Check sheet for the modelled part. Datum: model origin and axes. Units: mm. Face numbers are marked on the shaded views. A direction names the side the tool comes from. Give positions to 0.01 mm unless a question says otherwise; leave off trailing zeros. Order: outer loops, then holes, each group sorted by start corner. A loop starts at its lowest first (then second) coordinate and runs counter-clockwise, first axis right, second up.
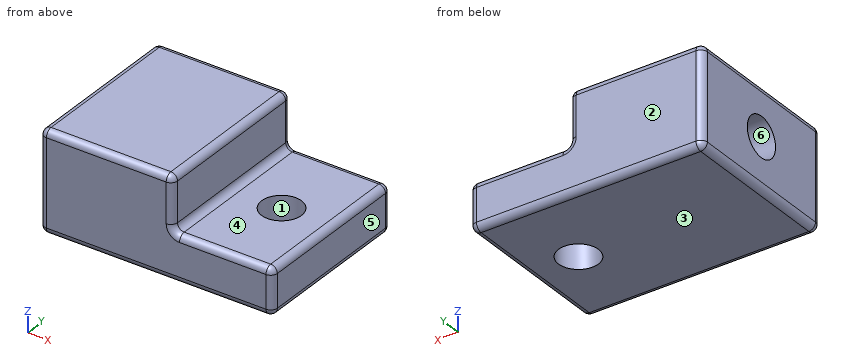
Autodesk Inventor part; units mm, degrees
ref_plane "YZ Plane" through (0, 0, 0) normal (1, 0, 0) x (0, 1, 0)
ref_plane "XZ Plane" through (0, 0, 0) normal (0, 1, 0) x (-1, 0, 0)
ref_plane "XY Plane" through (0, 0, 0) normal (0, 0, 1) x (1, 0, 0)
sketch "Boceto1" plane through (0, 0, 0) normal (0, 0, 1) x (1, 0, 0)
  line L0 (0, 0) -> (35, 0)
  line L1 (35, 0) -> (35, 25)
  line L2 (35, 25) -> (0, 25)
  line L3 (0, 25) -> (0, 0)
  dimension "d0" = 35
  dimension "d1" = 25
extrude "Extrusión1" add sketch "Boceto1" along normal blind 15
sketch "Boceto2" plane through (0, 0, 15) normal (0, 0, 1) x (1, 0, 0)
  line L0 (35, 0) -> (35, 25)
  line L1 (35, 25) -> (0, 25)
  line L2 (35, 0) -> (20, 0)
  line L3 (20, 0) -> (20, 25)
  line L4 (20, 25) -> (35, 25)
  line L5 (35, 25) -> (35, 0)
  point P0 (0, 0)
  dimension "d4" = 15
extrude "Extrusión2" cut sketch "Boceto2" against normal blind 8
fillet "Empalme1" radius 1 18 edges at (20, 25, 11) (20, 12.5, 15) (27.5, 25, 7) (20, 12.5, 7) (35, 12.5, 7) (35, 25, 3.5) (35, 12.5, 0) (17.5, 25, 0) (10, 25, 15) (0, 25, 7.5) (0, 12.5, 15) (10, 0, 15) (20, 0, 11) (27.5, 0, 7) (35, 0, 3.5) (17.5, 0, 0) (0, 0, 7.5) (0, 12.5, 0)
sketch "Boceto3" plane through (0, 0, 7) normal (0, 0, 1) x (1, 0, 0)
  point P0 (0, 0)
sketch "Boceto4" plane through (0, 0, 7) normal (0, 0, 1) x (1, 0, 0)
  line L0 (21, 24) -> (34, 24)
  line L1 (27.5, 24) -> (27.5, 12.5)
  line L2 (27.5, 12.5) -> (34, 12.5)
  circle A0 centre (27.5, 12.5) radius 3
  point P0 (0, 0)
  dimension "d8" = 11.5
  dimension "d9" = 6
sketch "Boceto5" plane through (0, 0, 7) normal (0, 0, 1) x (1, 0, 0)
  point P0 (0, 0)
extrude "Extrusión3" cut sketch "Boceto4" against normal blind 8
sketch "Boceto6" plane through (0, 1, 1) normal (-1, 0, 0) x (0, 0, 1)
  line L0 (13, 0) -> (13, 23)
  line L1 (13, 11.5) -> (6.5, 11.5)
  circle A0 centre (6.5, 11.5) radius 3
  point P0 (-1, -1)
  dimension "d12" = 6.5
  dimension "d13" = 6
extrude "Extrusión4" cut sketch "Boceto6" against normal blind 10
sketch "Boceto7" plane through (0, 1, 1) normal (-1, 0, 0) x (0, 0, 1)
  point P0 (-1, -1)
properties part number "Holder"
(1) Tool access check on the marked faces 4, 5 and 6. Record the directions out of +Z, -Z, +X, -X, +Y, -Y that give a thin tool (end or side, any length) a straight path to the whole face; none if there is none.
(2) Go/stop test with flat-tipped pins: P1, Ø1.5, axis at x = 22.5, z = 9, coming from the +Y side; P2, Ø6.5, axis at x = 30.5, y = 8.5, coming from the +Z side; P3, Ø1.8, axis at y = 14, z = 8, coming from the -X side; P4, Ø1.8, axis at y = 16, z = 11, coming from the +X side. Record where each tip stops, or that it passes through.
(3) Sectioned sample at B-B (x = 27.5). Enter the section's corners in (y, z).
(4) Thickness scan on L1, parallel to X at y = 12.5, z = 4.75; L2, parallel to X at y = 12.5, z = 1.5; L3, parallel to Y at x = 3.75, z = 7.5. Record the ranges inside material, lowest first.
(5) Sectioned sample at D-D (y = 6.75). Enter the section's corners in (x, z), plus the area to 3 significant figures.
(6) Release check for a two-part mould opening along Y. For the marked faces 1, 2 and 3 record: released by +Y, released by -Y, zero draft, split by the parting line, or undercut.
(7) Sectioned sample at A-A (y = 12.5). Enter the section's corners in (x, z), plus the area to 3 significant figures.
(8) Sectioned sample at C-C (z = 3.5). Enter the section's corners in (x, y), plus the area to 3 significant figures.
Values follow:
1. face 4: +Z, +X, +Y, -Y
1. face 5: +Z, -Z, +X, +Y, -Y
1. face 6: -X
2. P1: passes through
2. P2: stops at z = 7
2. P3: stops at x = 10
2. P4: stops at x = 20
3. outline: (0, 1) arc R1 ccw to (1, 0) - (9.5, 0) - (9.5, 7) - (1, 7) arc R1 ccw to (0, 6) - close; (15.5, 0) - (24, 0) arc R1 ccw to (25, 1) - (25, 6) arc R1 ccw to (24, 7) - (15.5, 7) - close
4. L1: x = 10 to 24.5, 30.5 to 35
4. L2: x = 0 to 24.5, 30.5 to 35
4. L3: y = 0 to 9.5, 15.5 to 25
5. outline: (0, 1) arc R1 ccw to (1, 0) - (34, 0) arc R1 ccw to (35, 1) - (35, 6) arc R1 ccw to (34, 7) - (21, 7) arc R1 cw to (20, 8) - (20, 14) arc R1 ccw to (19, 15) - (1, 15) arc R1 ccw to (0, 14) - close
5. area: 404 mm2
6. face 1: undercut
6. face 2: released by +Y
6. face 3: zero draft
7. outline: (0, 1) arc R1 ccw to (1, 0) - (24.5, 0) - (24.5, 7) - (21, 7) arc R1 cw to (20, 8) - (20, 14) arc R1 ccw to (19, 15) - (1, 15) arc R1 ccw to (0, 14) - (0, 10.5) - (10, 10.5) - (10, 4.5) - (0, 4.5) - close; (30.5, 0) - (34, 0) arc R1 ccw to (35, 1) - (35, 6) arc R1 ccw to (34, 7) - (30.5, 7) - close
7. area: 302 mm2
8. outline: (0, 1) arc R1 ccw to (1, 0) - (34, 0) arc R1 ccw to (35, 1) - (35, 24) arc R1 ccw to (34, 25) - (1, 25) arc R1 ccw to (0, 24) - close; hole circle Ø6 at (27.5, 12.5)
8. area: 846 mm2
